Design review of the part built by this model. Coordinates are the model's own, in mm. Face numbers are marked on the shaded views. A direction names the side the tool comes from. Give positions to 0.01 mm unless a question says otherwise; leave off trailing zeros. Loops run counter-clockwise (first coordinate to the right, second up) from the corner with the lowest first, then second, coordinate; pieces in that order, holes last. Notation, with made-up numbers: (45.5, 88) -> (59.5, 88) arc R31 cw to (59.5, 127) -> close; hole circle Ø8 at (80.5, 20.5). An arc over 180 degrees is marked (long way). Answer as CSV lines item,"result".
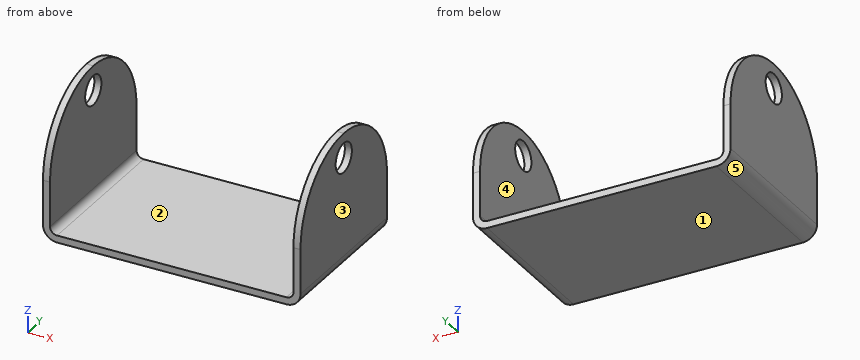
from build123d import *

# Parameters (mm, degrees)
F1_DEPTH = 25.4
F2_R     = 4.7625
F3_DEPTH = 83.567


with BuildPart() as f1:
    # F0 (on Front) → F1 (new body, symmetric)
    with BuildSketch(Plane.XZ):
        with BuildLine():
            ThreePointArc((-41.783, 4.572), (-40.443892, 1.339108), (-37.211, 0))
            Line((-37.211, 0), (37.211, 0))
            ThreePointArc((37.211, 0), (40.443892, 1.339108), (41.783, 4.572))
            Line((41.783, 4.572), (41.783, 44.45))
            Line((41.783, 44.45), (39.497, 44.45))
            Line((39.497, 44.45), (39.497, 4.572))
            ThreePointArc((39.497, 4.572), (38.827446, 2.955554), (37.211, 2.286))
            Line((37.211, 2.286), (-37.211, 2.286))
            ThreePointArc((-37.211, 2.286), (-38.827446, 2.955554), (-39.497, 4.572))
            Line((-39.497, 4.572), (-39.497, 44.45))
            Line((-39.497, 44.45), (-41.783, 44.45))
            Line((-41.783, 44.45), (-41.783, 4.572))
        make_face()
    extrude(amount=F1_DEPTH, both=True)

    # F2 (on face) → F3 (cut, through all)
    with BuildSketch(Plane(origin=(-41.783, 0, 0), x_dir=(0, -1, 0), z_dir=(-1, 0, 0))):
        with BuildLine():
            ThreePointArc((-25.4, 19.05), (-17.960512, 37.010512), (0, 44.45))
            Line((0, 44.45), (-25.4, 44.45))
            Line((-25.4, 44.45), (-25.4, 19.05))
        make_face()
        with Locations((0, 36.5125)):
            Circle(F2_R)
        with BuildLine():
            ThreePointArc((0, 44.45), (17.960512, 37.010512), (25.4, 19.05))
            Line((25.4, 19.05), (25.4, 44.45))
            Line((25.4, 44.45), (0, 44.45))
        make_face()
    extrude(amount=-F3_DEPTH, mode=Mode.SUBTRACT)


solid = f1.part
Q1. For the marked faces 1 and 2, list the 3-axis set-ups (+Z, -Z, +X, -X, +Y, -Y) from which the entire face can be reached by the end or side of a thin tool; tool diameter is ignored.
Filled sheet:
face 1,"-Z, +X, -X, +Y, -Y"
face 2,"+Z, +Y, -Y"
Q2. We need section B-B, the plane y = -18.5. State the section outline as (x, z) points, and give its area (3 significant figures).
Filled sheet:
outline,"(-41.78, 4.57) arc R4.57 ccw to (-37.21, 0) -> (37.21, 0) arc R4.57 ccw to (41.78, 4.57) -> (41.78, 36.45) -> (39.5, 36.45) -> (39.5, 4.57) arc R2.29 cw to (37.21, 2.29) -> (-37.21, 2.29) arc R2.29 cw to (-39.5, 4.57) -> (-39.5, 36.45) -> (-41.78, 36.45) -> close"
area,"341 mm^2"
Q3. The part is to be moulded in two halves that separate along X. For the marked faces 3, 4 and 5, say which applies: pulls with the +X half, pulls with the -X half, needs draft (parallel to the pull), parting line crosses it, or undercut.
Filled sheet:
face 3,"pulls with the +X half"
face 4,"undercut"
face 5,"pulls with the -X half"
Q4. We need section A-A, the plane z = 12. State the section outline as (x, y) points.
Filled sheet:
outline,"(-41.78, -25.4) -> (-39.5, -25.4) -> (-39.5, 25.4) -> (-41.78, 25.4) -> close; (39.5, -25.4) -> (41.78, -25.4) -> (41.78, 25.4) -> (39.5, 25.4) -> close"
Q5. Clearance check with a flat-ended pin moving along its axis: pin 1 Ø2 at (x, y) = (-16, 3.5) entering from +Z. State where the tip first meets the part, or that it passes through.
Filled sheet:
pin 1,"stops at z = 2.29"
Q6. We need section C-C, the plane z = 37.5. State the section outline as (x, y) points, and give its area (3 significant figures).
Filled sheet:
outline,"(-41.78, -17.46) -> (-39.5, -17.46) -> (-39.5, -4.66) -> (-41.78, -4.66) -> close; (-41.78, 4.66) -> (-39.5, 4.66) -> (-39.5, 17.46) -> (-41.78, 17.46) -> close; (39.5, -17.46) -> (41.78, -17.46) -> (41.78, -4.66) -> (39.5, -4.66) -> close; (39.5, 4.66) -> (41.78, 4.66) -> (41.78, 17.46) -> (39.5, 17.46) -> close"
area,"117 mm^2"
Q7. We need section D-D, the plane x = 34. State the section outline as (y, z) points.
Filled sheet:
outline,"(-25.4, 0) -> (25.4, 0) -> (25.4, 2.29) -> (-25.4, 2.29) -> close"
Q8. To check wall thickness, follow probe 1 along X at (y, z) = (-7.5, 18); probe 2 along Z at (x, y) = (-30, 1.5); probe 3 along Z at (x, y) = (40, 0) (3 decimals). State the ranges of each line that lie inside material, in increasing order. Write a range as from..to.
Filled sheet:
probe 1,"x = -41.78..-39.5, 39.5..41.78"
probe 2,"z = 0..2.29"
probe 3,"z = 0.949..31.75, 41.275..44.45"
